```python
from build123d import *

# Parameters (mm, degrees)
SKETCH_R  = 1
PAD_DEPTH = 6.8


with BuildPart() as part:
    # Sketch → Pad (new body)
    with BuildSketch(Plane.XY):
        with BuildLine():
            Line((0, 2.5), (-10, 2.5))
            Line((-10, 2.5), (-10, 1))
            Line((-7.365431, 1), (-10, 1))
            ThreePointArc((-1.938281, -1.578944), (-4.361066, 0.322469), (-7.365431, 1))
            ThreePointArc((-1.938281, -1.578944), (2.258026, -1.072996), (0, 2.5))
        make_face()
        Circle(SKETCH_R, mode=Mode.SUBTRACT)
    extrude(amount=PAD_DEPTH)


solid = part.part
```
Source: CAD feature listing. Evaluate the final solid. Frame: model axes, mm. A direction names the side the tool comes from. Round coordinates to 2 decimals unless told otherwise and drop trailing zeros. Loops run counter-clockwise (first coordinate to the right, second up) from the corner with the lowest first, then second, coordinate; pieces in that order, holes last. Notation, with made-up numbers: (28, 37) - (80, 37) arc R15 ccw to (80, 47) - close; hole circle Ø8 at (55, -18). An arc over 180 degrees is marked (long way). Use CSV: the item, a comma, the result in double quotes.
Q1. Reachability of faces 4 (the flat face through (-5, 2.5, 3)), 5 (the flat face through (-9, 1, 3)) from +Z, -Z, +X, -X, +Y, -Y: full face, straight path, thin tool, end or side. Return the list, or none.
Reported:
face 4,"+Z, -Z, +X, -X, +Y"
face 5,"+Z, -Z, -X, -Y"
Q2. Pin query (flat end, axial travel): pin 1 Ø0.8 at (x, z) = (-8, 2) entering from -Y; pin 2 Ø4 at (x, z) = (-8, 1.5) entering from -Y. Return the tip coordinate at first contact, or that it passes through.
Reported:
pin 1,"y = 1"
pin 2,"y = 0.87"
Q3. Mould query, pull axis X, two halves, no side actions, for faces 1 (the flat face through (-10, 2, 3)), 2 (the cylindrical face through (0, -1, 3)), 3 (the flat face through (-2, 1, 6.8)). Classes: pulls with the +X half, pulls with the -X half, needs draft (parallel to the pull), parting line crosses it, or undercut.
Reported:
face 1,"pulls with the -X half"
face 2,"undercut"
face 3,"needs draft"
Q4. Section query A-A, the plane z = 0.75. Output: boundary loops of the cut face in (x, y).
Reported:
outline,"(-10, 1) - (-7.37, 1) arc R7 cw to (-1.94, -1.58) arc R2.5 ccw (long way) to (0, 2.5) - (-10, 2.5) - close; hole circle Ø2 at (0, 0)"
Q5. Section query D-D, the plane x = -4. Output: boundary loops of the cut face in (y, z), then the cut area to 3 significant figures.
Reported:
outline,"(0.14, 0) - (2.5, 0) - (2.5, 6.8) - (0.14, 6.8) - close"
area,"16.1 mm^2"
Q6. Section query C-C, the plane x = 0.75. Output: boundary loops of the cut face in (y, z), then the cut area to 3 significant figures.
Reported:
outline,"(-2.38, 0) - (-0.66, 0) - (-0.66, 6.8) - (-2.38, 6.8) - close; (0.66, 0) - (2.38, 0) - (2.38, 6.8) - (0.66, 6.8) - close"
area,"23.4 mm^2"
Q7. Ray query, line 1 along Y through (x, z) = (0, 2.25); line 2 along Y through (x, z) = (-8.25, 3.5); line 3 along X through (y, z) = (0.25, 2.75). Return the intervals inside material, ascending.
Reported:
line 1,"-2.5 to -1, 1 to 2.5"
line 2,"1 to 2.5"
line 3,"-4.21 to -0.97, 0.97 to 2.49"
Q8. Section query B-B, the plane y = 0.2. Output: boundary loops of the cut face in (x, z).
Reported:
outline,"(-4.12, 0) - (-0.98, 0) - (-0.98, 6.8) - (-4.12, 6.8) - close; (0.98, 0) - (2.49, 0) - (2.49, 6.8) - (0.98, 6.8) - close"
